Here's how the part is built. I have some questions about the finished solid (model axes, mm). Face numbers are marked on the shaded views. A direction names the side the tool comes from. Give positions to 0.01 mm unless a question says otherwise; leave off trailing zeros. Write each loop counter-clockwise with the first axis right and the second up, starting at its lowest first coordinate (ties: lowest second). Pieces come first, ordered by that corner, then holes. Notation, with made-up numbers: (-6.5, 81.5) - (8.5, 81.5) arc R20 ccw to (8.5, 93.5) - close; hole circle Ø5 at (16, -13.75). An arc over 180 degrees is marked (long way). Use a Markdown table: item, result.
```python
from build123d import *

# Parameters (mm, degrees)
BOSS_EXTRUDE1_DEPTH     = 14
FILLET1_R               = 5
FILLET2_R               = 5
CUT_EXTRUDE3_DEPTH      = 10
CUT_EXTRUDE3_DEPTH_BACK = 10
SKETCH2_R               = 1.636049027
SKETCH4_W               = 29
SKETCH4_H               = 5
BOSS_EXTRUDE2_DEPTH     = 10
SKETCH5_R               = 2.3
CUT_EXTRUDE4_DEPTH      = 30
FILLET3_R               = 5


with BuildPart() as part:
    # Sketch1 → Boss-Extrude1 (new body)
    with BuildSketch(Plane.XY):
        Polygon((-24.5, 0), (-24.5, 5), (-14.5, 5), (-14.5, 44), (14.5, 44), (14.5, 5), (24.5, 5), (24.5, 0), (10, 0), (10, 39), (-10, 39), (-10, 0), align=None)
    extrude(amount=BOSS_EXTRUDE1_DEPTH)

    # Fillet1
    fillet1_edges = [part.edges().sort_by_distance(p)[0] for p in [
        (-14.5, 44, 7),
        (14.5, 44, 7),
        (24.5, 5, 7),
        (-24.5, 5, 7),
        (14.5, 5, 7),
        (-14.5, 5, 7),
    ]]
    fillet(fillet1_edges, radius=FILLET1_R - 0.0001)  # a hair under: the kernel refuses the full size

    # Fillet2
    fillet2_edges = [part.edges().sort_by_distance(p)[0] for p in [
        (10, 39, 7),
        (-10, 39, 7),
    ]]
    fillet(fillet2_edges, radius=FILLET2_R)

    # Sketch2 → Cut-Extrude3 (cut, two sides: drawn at the far end of the back side and taken through both)
    with BuildSketch(Plane(origin=(0, 0, 0), x_dir=(1, 0, 0), z_dir=(0, 1, 0)).offset(-CUT_EXTRUDE3_DEPTH_BACK)):
        with Locations(Location((-20, -7.523321805, 0), (0, 0, 72.20487372))):
            Circle(SKETCH2_R)
        with Locations(Location((20, -7.523321805, 0), (0, 0, 107.795126278))):
            Circle(SKETCH2_R)
    extrude(amount=CUT_EXTRUDE3_DEPTH + CUT_EXTRUDE3_DEPTH_BACK, mode=Mode.SUBTRACT)

    # Sketch4 → Boss-Extrude2 (add)
    with BuildSketch(Plane.XY.offset(14)):
        with Locations((0, 26.5)):
            Rectangle(SKETCH4_W, SKETCH4_H)
    extrude(amount=BOSS_EXTRUDE2_DEPTH)

    # Sketch5 → Cut-Extrude4 (cut)
    with BuildSketch(Plane(origin=(0, 44, 0), x_dir=(1, 0, 0), z_dir=(0, 1, 0))):
        with Locations(Location((-5.477408827, -19.118067384, 0), (0, 0, 270))):
            Circle(SKETCH5_R)
        with Locations(Location((4.70575, -19.10149527, 0), (0, 0, 270))):
            Circle(SKETCH5_R)
    extrude(amount=-CUT_EXTRUDE4_DEPTH, mode=Mode.SUBTRACT)

    # Fillet3
    fillet3_edges = [part.edges().sort_by_distance(p)[0] for p in [
        (-14.5, 26.5, 24),
        (14.5, 26.5, 24),
    ]]
    fillet(fillet3_edges, radius=FILLET3_R)


solid = part.part
```
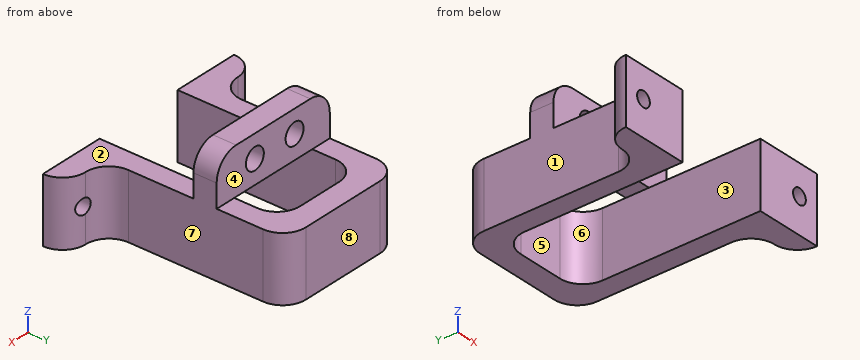
Item 1: Thinking about a two-plate mould opening in X: for the marked faces 6, 7 and 8, which applies, +X half, -X half, draft (parallel to the pull), parting line (faces both ways), or undercut?
Values:
| item | result |
|---|---|
| face 6 | undercut |
| face 7 | +X half |
| face 8 | draft |
Item 2: I need wall thicknesses on line 1 along Z through (x, y) = (-20, 2.3); line 2 along X through (y, z) = (15, 1.5); line 3 along Y through (x, z) = (-1, 5.75). Which ranges of each line are inside material? Lowest first, please. Write a range as [from, to].
Values:
| item | result |
|---|---|
| line 1 | z = [0, 5.89], [9.16, 14] |
| line 2 | x = [-14.5, -10], [10, 14.5] |
| line 3 | y = [39, 44] |
Item 3: If we section it at C-C, the plane x = -21: Write out the boundary of the cut face in (y, z), plus the area to 3 significant figures.
Values:
| item | result |
|---|---|
| outline | (0, 0) - (4.77, 0) - (4.77, 6.23) - (0, 6.23) - close; (0, 8.82) - (4.77, 8.82) - (4.77, 14) - (0, 14) - close |
| area | 54.4 mm2 |
Item 4: For the marked faces 1, 2, 3, 4 and 5, which set-ups out of +Z, -Z, +X, -X, +Y, -Y let a thin tool reach every point of the face, with its end or its side?
Values:
| item | result |
|---|---|
| face 1 | +Z, -Z, -X, +Y |
| face 2 | +Z, +X, -X, -Y |
| face 3 | -Z, -Y |
| face 4 | +Z, +X, -X, +Y |
| face 5 | +Z, -Z, -Y |
Item 5: If we section it at D-D, the plane z = 20.5: Write out the boundary of the cut face in (x, y).
Values:
| item | result |
|---|---|
| outline | (-14.27, 24) - (-7.32, 24) - (-7.32, 29) - (-14.27, 29) - close; (-3.64, 24) - (2.88, 24) - (2.88, 29) - (-3.64, 29) - close; (6.53, 24) - (14.27, 24) - (14.27, 29) - (6.53, 29) - close |
Item 6: Will these pins go through, and if not, where does the flat tip stop? pin 1 Ø9.5 at (y, z) = (29.5, 8) entering from -X; pin 2 Ø12 at (y, z) = (13.5, 21) entering from -X (3 decimals); pin 3 Ø12 at (y, z) = (9.5, 8) entering from +X; pin 4 Ø4.5 at (x, y) = (16, 10.5) entering from +Z.
Values:
| item | result |
|---|---|
| pin 1 | stops at x = -14.5 |
| pin 2 | passes through |
| pin 3 | stops at x = 23.07 |
| pin 4 | stops at z = 14 |
Item 7: If we section it at A-A, the plane y = 13: Write out the boundary of the cut face in (x, z).
Values:
| item | result |
|---|---|
| outline | (-14.5, 0) - (-10, 0) - (-10, 14) - (-14.5, 14) - close; (10, 0) - (14.5, 0) - (14.5, 14) - (10, 14) - close |
Item 8: If we section it at B-B, the plane z = 8.5: Count the separate pieces of the cut face and the enclosed holes in it, plus the area to 3 significant figures.
Values:
| item | result |
|---|---|
| separate pieces | 3 |
| enclosed holes | 0 |
| area | 570 mm2 |
